Input: part model. Units: mm. Frame: model coordinates. Face numbers are marked on the shaded views. A direction names the side the tool comes from. Give positions to 0.01 mm unless a question says otherwise; leave off trailing zeros. Write each loop counter-clockwise with the first axis right and the second up, starting at its lowest first coordinate (ties: lowest second). Pieces come first, ordered by that corner, then holes.
```python
from build123d import *

# Parameters (mm, degrees)
SKETCH1_W                            = 76.2
SKETCH1_H                            = 76.2
BOSS_EXTRUDE1_DEPTH                  = 6.35
SKETCH2_W                            = 38.1
SKETCH2_H                            = 38.1
BOSS_EXTRUDE2_DEPTH                  = 69.85
BOSS_EXTRUDE3_DEPTH                  = 95.25
BOSS_EXTRUDE4_START                  = 95.25
SKETCH2_5_W                          = 25.4
SKETCH2_5_H                          = 25.4
SKETCH2_5_R                          = 4.175
BOSS_EXTRUDE4_DEPTH                  = 6.35
BOSS_EXTRUDE6_START                  = 93.9
SKETCH2_7_R                          = 4.175
BOSS_EXTRUDE6_DEPTH                  = 1.35
BOSS_EXTRUDE6_DRAFT                  = -30
F_8_0_199_DIAMETER_HOLE1_D           = 5.0546
F_8_0_199_DIAMETER_HOLE1_DEPTH       = 8.89
F_8_0_199_DIAMETER_HOLE1_CSINK_D     = 6.3246
F_8_0_199_DIAMETER_HOLE1_CSINK_ANGLE = 90
F_8_0_199_DIAMETER_HOLE1_TIP         = 1.518555042
F_8_START                            = -31.75
F_8_CLEARANCE_SLOT1_DEPTH            = 63.5
FILLET2_R                            = 6.35
CHAMFER2_SIZE                        = 3.175
CHAMFER3_SIZE                        = 3.175
CHAMFER4_SIZE                        = 0.396875


with BuildPart() as part:
    # Sketch1 → Boss-Extrude1 (new body)
    with BuildSketch(Plane(origin=(0, 0, 0), x_dir=(1, 0, 0), z_dir=(0, 1, 0))):
        Rectangle(SKETCH1_W, SKETCH1_H)
    extrude(amount=BOSS_EXTRUDE1_DEPTH)

    # Sketch2 → Boss-Extrude2 (add)
    with BuildSketch(Plane(origin=(0, 0, 0), x_dir=(1, 0, 0), z_dir=(0, 1, 0))):
        Rectangle(SKETCH2_W, SKETCH2_H)
    extrude(amount=BOSS_EXTRUDE2_DEPTH)

    # Sketch2<3> → Boss-Extrude3 (add)
    with BuildSketch(Plane(origin=(0, 0, 0), x_dir=(1, 0, 0), z_dir=(0, 1, 0))):
        Polygon((-19.05, 19.05), (-19.05, -19.05), (19.05, -19.05), (19.05, -6.35), (-6.35, -6.35), (-6.35, 19.05), align=None)
    extrude(amount=BOSS_EXTRUDE3_DEPTH)

    # Sketch2<5> → Boss-Extrude4 (add)
    # profile 1 of 3: a face of its own
    with BuildSketch(Plane(origin=(0, 0, 0), x_dir=(1, 0, 0), z_dir=(0, 1, 0)).offset(BOSS_EXTRUDE4_START)):
        Polygon((-19.05, 19.05), (-19.05, -19.05), (19.05, -19.05), (19.05, -6.35), (-6.35, -6.35), (-6.35, 19.05), align=None)
    # profile 2 of 3: a face of its own
    with BuildSketch(Plane(origin=(0, 0, 0), x_dir=(1, 0, 0), z_dir=(0, 1, 0)).offset(BOSS_EXTRUDE4_START)):
        with Locations((6.35, 6.35)):
            Rectangle(SKETCH2_5_W, SKETCH2_5_H)
        with Locations((6.35, 6.35)):
            Circle(SKETCH2_5_R, mode=Mode.SUBTRACT)
    # profile 3 of 3: a face of its own
    with BuildSketch(Plane(origin=(0, 0, 0), x_dir=(1, 0, 0), z_dir=(0, 1, 0)).offset(BOSS_EXTRUDE4_START)):
        with Locations((6.35, 6.35)):
            Circle(SKETCH2_5_R)
    extrude(amount=BOSS_EXTRUDE4_DEPTH)

    # Boss-Extrude5: read off the stored shape, not the designer's step
    # Boss-Extrude5 outline → Boss-Extrude5 (revolve)
    with BuildSketch(Plane(origin=(6.35, 0, -6.35), x_dir=(1, 0, 0), z_dir=(0, 0, 1))):
        Polygon((4.175, 71.2), (0, 71.2), (0, 69.85), (4.954422863, 69.85), align=None)
    revolve(axis=Axis((6.35, 0, -6.35), (0, 1, 0)))


with BuildPart() as boss_extrude6_tool:
    # Sketch2<7> → Boss-Extrude6 (with draft: the straight prism first)
    with BuildSketch(Plane(origin=(0, 0, 0), x_dir=(1, 0, 0), z_dir=(0, 1, 0)).offset(BOSS_EXTRUDE6_START)):
        with Locations((6.35, 6.35)):
            Circle(SKETCH2_7_R)
    extrude(amount=BOSS_EXTRUDE6_DEPTH)
    # Boss-Extrude6: the draft: its side faces are tilted about the plane it starts from
    boss_extrude6_sides = [boss_extrude6_tool.faces().sort_by_distance(p)[0] for p in [
        (2.175, 94.575, -6.35),
    ]]
    draft(boss_extrude6_sides, Plane(origin=(0, 0, 0), x_dir=(1, 0, 0), z_dir=(0, 1, 0)).offset(BOSS_EXTRUDE6_START), BOSS_EXTRUDE6_DRAFT)


with BuildPart() as part_1:
    add(part.part)

    # Boss-Extrude6: add boss_extrude6_tool
    add(boss_extrude6_tool.part)

    # #8 (0.199) Diameter Hole1
    with Locations(Plane(origin=(0, 71.2, 0), x_dir=(1, 0, 0), z_dir=(0, 1, 0))):
        with Locations((6.35, 6.35)):
            CounterSinkHole(F_8_0_199_DIAMETER_HOLE1_D / 2, F_8_0_199_DIAMETER_HOLE1_CSINK_D / 2, depth=F_8_0_199_DIAMETER_HOLE1_DEPTH, counter_sink_angle=F_8_0_199_DIAMETER_HOLE1_CSINK_ANGLE)
            with Locations((0, 0, -(F_8_0_199_DIAMETER_HOLE1_DEPTH + F_8_0_199_DIAMETER_HOLE1_TIP / 2))):  # 118° drill point
                Cone(0, F_8_0_199_DIAMETER_HOLE1_D / 2, F_8_0_199_DIAMETER_HOLE1_TIP, mode=Mode.SUBTRACT)

    # Sketch8 → M5 Clearance Hole1 (revolve, cut)
    with BuildSketch(Plane(origin=(6.35, 93.9, -6.35), x_dir=(0, 0, -1), z_dir=(1, 0, 0))):
        Polygon((0, 0), (0, 7.7), (3.5, 7.7), (2.75, 6.95), (2.75, 0.75), (3.5, 0), align=None)
    revolve(axis=Axis((6.35, 87.55, -6.35), (0, 1, 0)), mode=Mode.SUBTRACT)

    # #8 Clearance Slot1: read off the stored shape, not the designer's step
    # #8 Clearance Slot1 outline → #8 Clearance Slot1 (cut)
    with BuildSketch(Plane.XY.offset(F_8_START)):
        Polygon((34.6329, 6.35), (28.8671, 6.35), (29.5021, 5.715), (29.5021, 0.635), (28.8671, 0), (34.6329, 0), (33.9979, 0.635), (33.9979, 5.715), align=None)
        Polygon((-29.5021, 5.715), (-28.8671, 6.35), (-34.6329, 6.35), (-33.9979, 5.715), (-33.9979, 0.635), (-34.6329, 0), (-28.8671, 0), (-29.5021, 0.635), align=None)
    extrude(amount=F_8_CLEARANCE_SLOT1_DEPTH, mode=Mode.SUBTRACT)

    # 8 Clearance Slot1 2 outline → 8 Clearance Slot1 2 (revolve, cut)
    with BuildSketch(Plane(origin=(31.75, 0, -31.75), x_dir=(1, 0, 0), z_dir=(0, 0, 1))):
        Polygon((0, 0), (2.8829, 0), (2.2479, 0.635), (2.2479, 5.715), (2.8829, 6.35), (0, 6.35), align=None)
    revolve(axis=Axis((31.75, 0, -31.75), (0, 1, 0)), mode=Mode.SUBTRACT)

    # 8 Clearance Slot1 3 outline → 8 Clearance Slot1 3 (revolve, cut)
    with BuildSketch(Plane(origin=(31.75, 0, 31.75), x_dir=(1, 0, 0), z_dir=(0, 0, 1))):
        Polygon((0, 0), (2.8829, 0), (2.2479, 0.635), (2.2479, 5.715), (2.8829, 6.35), (0, 6.35), align=None)
    revolve(axis=Axis((31.75, 0, 31.75), (0, 1, 0)), mode=Mode.SUBTRACT)

    # 8 Clearance Slot1 4 outline → 8 Clearance Slot1 4 (revolve, cut)
    with BuildSketch(Plane(origin=(-31.75, 0, -31.75), x_dir=(1, 0, 0), z_dir=(0, 0, 1))):
        Polygon((0, 0), (2.8829, 0), (2.2479, 0.635), (2.2479, 5.715), (2.8829, 6.35), (0, 6.35), align=None)
    revolve(axis=Axis((-31.75, 0, -31.75), (0, 1, 0)), mode=Mode.SUBTRACT)

    # 8 Clearance Slot1 5 outline → 8 Clearance Slot1 5 (revolve, cut)
    with BuildSketch(Plane(origin=(-31.75, 0, 31.75), x_dir=(1, 0, 0), z_dir=(0, 0, 1))):
        Polygon((0, 0), (2.8829, 0), (2.2479, 0.635), (2.2479, 5.715), (2.8829, 6.35), (0, 6.35), align=None)
    revolve(axis=Axis((-31.75, 0, 31.75), (0, 1, 0)), mode=Mode.SUBTRACT)

    # Fillet2
    fillet2_edges = [part_1.edges().sort_by_distance(p)[0] for p in [
        (19.05, 38.1, -19.05),
        (-19.05, 53.975, -19.05),
        (-19.05, 53.975, 19.05),
        (19.05, 53.975, 19.05),
        (-6.35, 82.55, 6.35),
        (19.05, 98.425, -19.05),
        (38.1, 3.175, 38.1),
        (-38.1, 3.175, 38.1),
        (-38.1, 3.175, -38.1),
        (38.1, 3.175, -38.1),
    ]]
    fillet(fillet2_edges, radius=FILLET2_R)

    # Chamfer2
    chamfer2_edges = [part_1.edges().sort_by_distance(p)[0] for p in [
        (-6.35, 69.85, -9.525),
        (9.525, 69.85, 6.35),
        (-4.490128061, 69.85, 4.490128061),
        (-4.490128061, 95.25, 4.490128061),
        (-19.05, 6.35, 0),
        (0, 6.35, -19.05),
        (19.05, 6.35, 0),
        (0, 6.35, 19.05),
        (-17.190128061, 6.35, -17.190128061),
        (17.190128061, 6.35, -17.190128061),
        (-17.190128061, 6.35, 17.190128061),
        (17.190128061, 6.35, 17.190128061),
        (-6.35, 95.25, -9.525),
        (9.525, 95.25, 6.35),
    ]]
    chamfer(chamfer2_edges, length=CHAMFER2_SIZE)

    # Chamfer3
    chamfer3_edges = [part_1.edges().sort_by_distance(p)[0] for p in [
        (17.190128061, 69.85, -17.190128061),
        (0, 101.6, -19.05),
        (19.05, 101.6, 0),
        (-19.05, 101.6, 0),
        (0, 101.6, 19.05),
        (17.190128061, 101.6, 17.190128061),
        (-17.190128061, 101.6, 17.190128061),
        (-17.190128061, 101.6, -17.190128061),
        (17.190128061, 101.6, -17.190128061),
        (19.05, 69.85, -4.7625),
        (4.7625, 69.85, -19.05),
    ]]
    chamfer(chamfer3_edges, length=CHAMFER3_SIZE)

    # Chamfer4
    chamfer4_edges = [part_1.edges().sort_by_distance(p)[0] for p in [
        (4.7625, 95.25, -19.05),
        (19.05, 95.25, -4.7625),
        (17.190128061, 95.25, -17.190128061),
        (-38.1, 0, 0),
        (-38.1, 6.35, 0),
        (38.1, 0, 0),
        (0, 0, 38.1),
        (0, 0, -38.1),
        (36.240128061, 0, -36.240128061),
        (36.240128061, 0, 36.240128061),
        (-36.240128061, 0, 36.240128061),
        (-36.240128061, 0, -36.240128061),
        (0, 6.35, -38.1),
        (38.1, 6.35, 0),
        (0, 6.35, 38.1),
        (36.240128061, 6.35, -36.240128061),
        (36.240128061, 6.35, 36.240128061),
        (-36.240128061, 6.35, 36.240128061),
        (-36.240128061, 6.35, -36.240128061),
    ]]
    chamfer(chamfer4_edges, length=CHAMFER4_SIZE)


solid = part_1.part
```
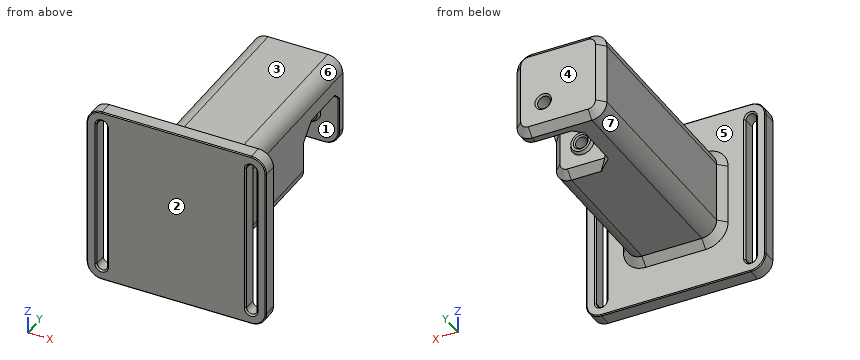
Item 1: Section A-A (y = 79). Return loops of the section in (x, z), and give its area (3 significant figures).
Item 2: Mould query, pull axis Y, two halves, no side actions, for the marked faces 1, 2, 3 and 4. Classes: +Y half, -Y half, draft (parallel to the pull), parting line (faces both ways), or undercut.
Item 3: Set-up query: the marked faces 5, 6 and 7. Return all of +Z, -Z, +X, -X, +Y, -Y with unobstructed straight access to the full face (end or side cutting, diameter ignored); none if empty.
Item 4: Pin query (flat end, axial travel): pin 1 (1.5 mm diameter, centred on x = -15.5, y = 62.5, fed in from -Z); pin 2 (1.5 mm diameter, centred on y = 47.5, z = 16, fed in from -X); pin 3 (7.5 mm diameter, centred on x = -3, y = 52.5, fed in from -Z). Return the tip coordinate at first contact, or that it passes through.
Item 5: Section B-B (y = 29.5). Return loops of the section in (x, z), and give its area (3 significant figures).
Item 6: Ray query, line 1 (X direction, y = 96.5, z = -6.35); line 2 (Z direction, x = 6.35, y = 66.5); line 3 (Z direction, x = 6, y = 84). Return the intervals inside material, ascending.
Solved:
1. outline: (-19.05, -12.7) arc R6.35 ccw to (-12.7, -19.05) - (-6.35, -19.05) - (-6.35, 0) arc R6.35 cw to (0, 6.35) - (19.05, 6.35) - (19.05, 12.7) arc R6.35 ccw to (12.7, 19.05) - (-12.7, 19.05) arc R6.35 ccw to (-19.05, 12.7) - close
1. area: 789 mm2
2. face 1: undercut
2. face 2: -Y half
2. face 3: draft
2. face 4: +Y half
3. face 5: +Y
3. face 6: +Z, +X, +Y
3. face 7: -Z, -X, +Y
4. pin 1: stops at z = -18.71
4. pin 2: stops at x = -18.52
4. pin 3: stops at z = -19.05
5. outline: (-19.05, -12.7) arc R6.35 ccw to (-12.7, -19.05) - (12.7, -19.05) arc R6.35 ccw to (19.05, -12.7) - (19.05, 12.7) arc R6.35 ccw to (12.7, 19.05) - (-12.7, 19.05) arc R6.35 ccw to (-19.05, 12.7) - close
5. area: 1,420 mm2
6. line 1: x = -19.05 to 3.6, 9.1 to 19.05
6. line 2: z = -19.05 to -8.88, -3.82 to 19.05
6. line 3: z = 6.35 to 19.05
